The model under review builds one solid part; all positions refer to its coordinate system, in mm. Coordinates: 2 decimals unless noted, no trailing zeros. Loops run counter-clockwise (first coordinate to the right, second up) from the corner with the lowest first, then second, coordinate; pieces in that order, holes last. Notation, with made-up numbers: M 84.25,-33 L 112.25,-33 A30 ccw 112.25,5 Z; hole C 39,48 d10. An arc over 180 degrees is marked long. Use one line per item in the form item = value.
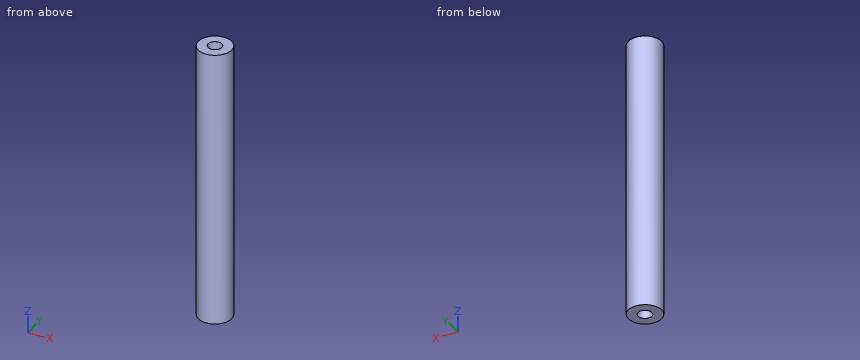
```python
from build123d import *

# Parameters (mm, degrees)
SKETCH_1_R             = 6
EXTRUDE_1_DEPTH        = 100
HOLE_WIZARD_M6_1_D     = 5
HOLE_WIZARD_M6_1_DEPTH = 15
HOLE_WIZARD_M6_1_TIP   = 1.502151548
HOLE_WIZARD_M6_2_D     = 5
HOLE_WIZARD_M6_2_DEPTH = 15
HOLE_WIZARD_M6_2_TIP   = 1.502151548


with BuildPart() as part:
    # 草图1 → 凸台-拉伸1 (new body)
    with BuildSketch(Plane.XY):
        Circle(SKETCH_1_R)
    extrude(amount=EXTRUDE_1_DEPTH)

    # M6 螺纹孔1
    with Locations(Plane(origin=(0, 0, 0), x_dir=(-1, 0, 0), z_dir=(0, 0, -1))):
        with Locations((0, 0)):
            Hole(HOLE_WIZARD_M6_1_D / 2, depth=HOLE_WIZARD_M6_1_DEPTH)
            with Locations((0, 0, -(HOLE_WIZARD_M6_1_DEPTH + HOLE_WIZARD_M6_1_TIP / 2))):  # 118° drill point
                Cone(0, HOLE_WIZARD_M6_1_D / 2, HOLE_WIZARD_M6_1_TIP, mode=Mode.SUBTRACT)

    # M6 螺纹孔2
    with Locations(Plane.XY.offset(100)):
        with Locations((0, 0)):
            Hole(HOLE_WIZARD_M6_2_D / 2, depth=HOLE_WIZARD_M6_2_DEPTH)
            with Locations((0, 0, -(HOLE_WIZARD_M6_2_DEPTH + HOLE_WIZARD_M6_2_TIP / 2))):  # 118° drill point
                Cone(0, HOLE_WIZARD_M6_2_D / 2, HOLE_WIZARD_M6_2_TIP, mode=Mode.SUBTRACT)


solid = part.part
```
1. Add section B-B (z = 21). State the section outline as (x, y) points.
Response values:
outline = C 0,0 d12
2. Add section A-A (y = -4). State the section outline as (x, z) points.
Response values:
outline = M -4.47,0 L 4.47,0 L 4.47,100 L -4.47,100 Z
3. Insertion check: P1, Ø6, axis at x = 2.5, z = 41, coming from the +Y side; P2, Ø3, axis at x = -4, z = 29, coming from the -Y side; P3, Ø4.5, axis at x = 0, y = 0, coming from the -Z side; P4, Ø4, axis at x = 0, y = 0, coming from the +Z side. Each pin has a flat end and moves straight along its axis. Give the tip position at first contact, or say it passes through.
Response values:
P1 = 6
P2 = -5.45
P3 = 15.15
P4 = 84.7
4. Wall thickness on line 1 along Y through (x, z) = (0, 93.5); line 2 along Y through (x, z) = (-0.5, 87); line 3 along X through (y, z) = (-3.75, 74): over which ranges is each line inside the solid? List them lowest first. Write a range as from..to.
Response values:
line_1 = -6..-2.5, 2.5..6
line_2 = -5.98..-2.45, 2.45..5.98
line_3 = -4.68..4.68
